Autodesk Inventor part; units mm, degrees
ref_plane "YZ Plane" through (0, 0, 0) normal (1, 0, 0) x (0, 1, 0)
ref_plane "XZ Plane" through (0, 0, 0) normal (0, 1, 0) x (-1, 0, 0)
ref_plane "XY Plane" through (0, 0, 0) normal (0, 0, 1) x (1, 0, 0)
sketch "Sketch1" plane through (0, 0, 0) normal (0, 1, 0) x (-1, 0, 0)
  line L0 (0, 8.25) -> (0, -8.25) construction
  line L1 (-2.5, 8.25) -> (-2.5, -8.25)
  line L2 (2.5, -8.25) -> (2.5, 8.25)
  arc A0 (2.5, 8.25) -> (-2.5, 8.25) centre (0, 8.25) ccw
  arc A1 (-2.5, -8.25) -> (2.5, -8.25) centre (0, -8.25) ccw
  circle A2 centre (0, 8.25) radius 2.1
  circle A3 centre (0, -8.25) radius 2.1
  line L3 (2.5, 13.25) -> (-2.5, 13.25)
  line L4 (-2.5, 13.25) -> (-2.5, 3.25)
  line L5 (-2.5, 3.25) -> (2.5, 3.25)
  line L6 (2.5, 3.25) -> (2.5, 13.25)
  line L7 (2.5, 13.25) -> (-2.5, 3.25) construction
  line L8 (-2.5, 13.25) -> (2.5, 3.25) construction
  line L9 (0, 8.25) -> (0, -35.75)
  circle A4 centre (0, -35.75) radius 27.5
  line L10 (-6.2348, -8.9661) -> (-2.5, 3.25)
  line L11 (2.5, 3.25) -> (6.2348, -8.9661)
  line L12 (3.5, 13.25) -> (-3.5, 13.25)
  line L13 (-3.5, 13.25) -> (-3.5, 3.25)
  line L14 (-3.5, 3.25) -> (3.5, 3.25)
  line L15 (3.5, 3.25) -> (3.5, 13.25)
  line L16 (3.5, 13.25) -> (-3.5, 3.25) construction
  line L17 (-3.5, 13.25) -> (3.5, 3.25) construction
  point P0 (0, 0)
  point P1 (-2.5, 8.25)
  point P2 (2.5, 8.25)
  point P3 (2.5, 3.25)
  point P4 (2.4974, -8.3636)
  point P5 (-2.4974, -8.3636)
  point P6 (2.5, 3.25)
  point P7 (-2.5, 3.25)
  point P8 (-2.5, 13.25)
  dimension "d1" = 2.5
  dimension "d2" = 4.2
  dimension "d6" = 10
  dimension "d7" = 16.5
  dimension "d8" = 44
  dimension "d9" = 17
  dimension "d12" = 10
  dimension "d13" = 7
extrude "Extrusion1" add sketch "Sketch1" along normal blind 5 contours A0 L2 L5 L1 | L4 L3 L6 A0 | L1 L14 L13 L12 L4 | L5 L9 A3 A4 A1 L1 | L1 A1 A4 L10 | L6 L12 L15 L14 L2 | L5 L2 A1 A4 A3 L9 | L11 A4 A1 L2 | A4 A3 L9 A1 | L9 A4 A3 | A3 A4 L9 | L9 A3 A4 A1 | A4 L9 A3 | A4 A3 L9
fillet "Fillet2" radius 0.5 2 edges at (6.2348, 2.5, -8.9661) (-6.2348, 2.5, -8.9661)
fillet "Fillet4" radius 4.75 4 edges at (3.5, 2.5, 3.25) (2.5, 2.5, 3.25) (-3.5, 2.5, 3.25) (-2.5, 2.5, 3.25)
fillet "Fillet5" radius 1 2 edges at (-3.5, 2.5, 13.25) (3.5, 2.5, 13.25)
equation "\"d12\" = d6"
properties part number "11_Chot_banh_lai"
Design review of the part built by this model. Coordinates are the model's own, in mm. A direction names the side the tool comes from. Coordinates: 2 decimals unless noted, no trailing zeros. Order: outer loops, then holes, each group sorted by start corner. A loop starts at its lowest first (then second) coordinate and runs counter-clockwise, first axis right, second up. Notation, with made-up numbers: (60, 4) -> (69, 4) arc R18 ccw to (69, 10) -> close; hole circle Ø7 at (34, 50). An arc over 180 degrees is marked (long way). Use one line per item in the form item = value. Start each with the question number.
(1) Insertion check: pin 1 (2 mm diameter, centred on x = -4, y = 3, fed in from -Z); pin 2 (6.5 mm diameter, centred on x = 0, z = 8.25, fed in from -Y); pin 3 (1.5 mm diameter, centred on y = 3.5, z = 9, fed in from +X). Each pin has a flat end and moves straight along its axis. Give the tip position at first contact, or say it passes through.
(2) Add section A-A on x = 0. State the section outline as (y, z) points.
(3) For probe 1 along X at (y, z) = (1.6, 8.25); probe 2 along Z at (x, y) = (0, 3.45); probe 3 along X at (y, z) = (0.5, 7.5), list the stretches that pass through material, from the lowest coordinate up.
(4) Add section C-C on z = 8.25. State the section outline as (x, y) points.
(5) For faces 1 (the cylindrical face through (3.98, 2.46, -8.54)), 2 (the flat face through (3.5, 2, 9)), 3 (the flat face through (-3.5, 2, 9)), list the 3-axis set-ups (+Z, -Z, +X, -X, +Y, -Y) from which the entire face can be reached by the end or side of a thin tool; tool diameter is ignored.
(6) Add section B-B on y = 2.3. State the section outline as (x, z) points, plus the area to 3 significant figures.
(7) Add section D-D on z = 2.25. State the section outline as (x, y) points.
(8) The part is to be moulded in two halves that separate along Z. For faces 4 (the cylindrical face through (-0.05, 2.46, -10.75)), 5 (the flat face through (0, 0, -1)), 6 (the cylindrical face through (0.273, 2.465, 6.168)), say which applies: +Z half, -Z half, draft (parallel to the pull), parting line (faces both ways), or undercut.
Answer block:
q1.pin_1 = -8.71
q1.pin_2 = 0
q1.pin_3 = 3.5
q2.outline = (0, -10.75) -> (5, -10.75) -> (5, 6.15) -> (0, 6.15) -> close; (0, 10.35) -> (5, 10.35) -> (5, 13.25) -> (0, 13.25) -> close
q3.probe_1 = -3.5 to -2.1, 2.1 to 3.5
q3.probe_2 = -10.75 to 6.15, 10.35 to 13.25
q3.probe_3 = -3.5 to -1.96, 1.96 to 3.5
q4.outline = (-3.5, 0) -> (-2.1, 0) -> (-2.1, 5) -> (-3.5, 5) -> close; (2.1, 0) -> (3.5, 0) -> (3.5, 5) -> (2.1, 5) -> close
q5.face_1 = -Z, +Y, -Y
q5.face_2 = +Z, +X, +Y, -Y
q5.face_3 = +Z, -X, +Y, -Y
q6.outline = (-5.99, -8.15) arc R0.5 ccw to (-5.41, -8.79) arc R27.5 cw to (-2.5, -8.36) arc R2.5 ccw to (2.5, -8.36) arc R27.5 cw to (5.41, -8.79) arc R0.5 ccw to (5.99, -8.15) -> (3.08, 1.37) arc R4.75 cw to (3.18, 4.46) arc R4.75 ccw to (3.5, 6.17) -> (3.5, 12.25) arc R1 ccw to (2.5, 13.25) -> (-2.5, 13.25) arc R1 ccw to (-3.5, 12.25) -> (-3.5, 6.17) arc R4.75 ccw to (-3.18, 4.46) arc R4.75 cw to (-3.08, 1.37) -> close; hole circle Ø4.2 at (0, 8.25)
q6.area = 165 mm²
q7.outline = (-2.89, 0) -> (2.89, 0) -> (2.89, 5) -> (-2.89, 5) -> close
q8.face_4 = -Z half
q8.face_5 = draft
q8.face_6 = undercut
